Can you work these out from the model? Positions are in its coordinate system, mm. Face numbers are marked on the shaded views. A direction names the side the tool comes from. Give positions to 0.01 mm unless a question says otherwise; leave off trailing zeros. Loops run counter-clockwise (first coordinate to the right, second up) from the corner with the lowest first, then second, coordinate; pieces in that order, holes last. Notation, with made-up numbers: (37, 3.5) - (84, 3.5) arc R25 cw to (84, 27.5) - close; hole circle Ø2 at (77, 54). An arc over 180 degrees is marked (long way). Answer as a JSON object with one key per item and string values. Group by question number.
Item 1: Please list where these lines run through material, in increasing order: L1, parallel to Z at x = 0, y = 1; L2, parallel to X at y = -0.5, z = 1.
Item 2: Which directions (+Z, -Z, +X, -X, +Y, -Y) give clear straight access to the entire face, cutting with the end or side of a thin tool? Please do the marked faces 1 and 2.
Item 3: Suppose I cut it at C-C on y = 12. Write out the boundary of the cut face in (x, z), and give its area (3 significant figures).
Item 4: Will these pins go through, and if not, where does the flat tip stop? pin 1 (2 mm diameter, centred on y = 5, z = -2, fed in from -X); pin 2 (2 mm diameter, centred on y = 6, z = 1.5, fed in from +X); pin 3 (1 mm diameter, centred on x = 1.5, z = -2, fed in from -Y).
Item 5: Suppose I cut it at A-A on y = 7.75. Write out the boundary of the cut face in (x, z), and give its area (3 significant figures).
Item 6: Suppose I cut it at B-B on y = -6.75. Write out the boundary of the cut face in (x, z).
Item 7: Thinking about a two-plate mould opening in Z: for the marked faces 3, 4 and 5, which applies, pulls with the +Z half, pulls with the -Z half, needs draft (parallel to the pull), parting line crosses it, or undercut?
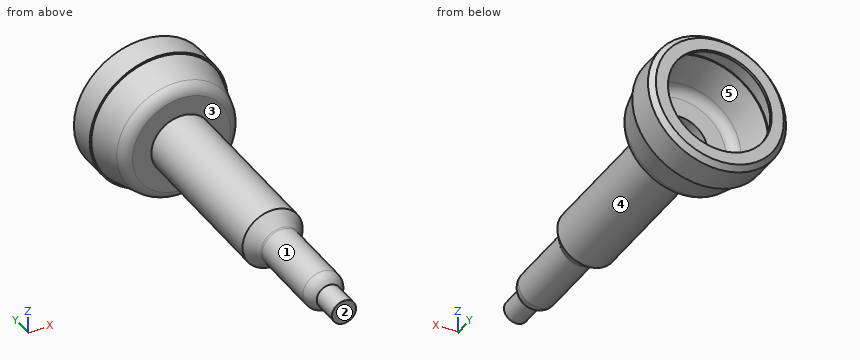
from build123d import *

# Parameters (mm, degrees)
BOSS_EXTRUDE1_DEPTH      = 7
BOSS_EXTRUDE1_DEPTH_BACK = 5
SKETCH2_R                = 1.4
SKETCH3_OUTSIDE_W        = 18.066
SKETCH3_OUTSIDE_H        = 18.066
SKETCH3_OUTSIDE_R        = 0.875
CUT_EXTRUDE1_DEPTH       = 2
FILLET1_R                = 1


with BuildPart() as part:
    # Sketch1 → Revolve2 (revolve)
    with BuildSketch(Plane.XY):
        with BuildLine():
            Line((-3.755778652, 14.546362803), (-4.55, 14.546362803))
            Line((-4.55, 14.546362803), (-4.8, 14.296362803))
            Line((-4.8, 14.296362803), (-4.8, 12.499997602))
            Line((-4.8, 12.499997602), (-4.726187471, 12.499997602))
            Line((-4.726187471, 12.499997602), (-4.085093395, 10.107402835))
            ThreePointArc((-4.085093395, 10.107402835), (-3.828996553, 9.665101687), (-3.348994918, 9.489561582))
            Line((-3.348994918, 9.489561582), (-2, 9.489561582))
            Line((-2, 9.489561582), (-2, -2.631922723))
            Line((-2, -2.631922723), (-1.256169591, -3.694222639))
            ThreePointArc((-1.256169591, -3.694222639), (-1.22925661, -3.748796766), (-1.22, -3.808937926))
            Line((-1.22, -3.808937926), (-1.22, -4.710135178))
            ThreePointArc((-1.22, -4.710135178), (-1.161421356, -4.851556534), (-1.02, -4.910135178))
            Line((-1.02, -4.910135178), (0, -4.910135178))
            Line((0, -4.910135178), (0, -5.090135178))
            Line((0, -5.090135178), (-1.2, -5.090135178))
            ThreePointArc((-1.2, -5.090135178), (-1.341421356, -5.031556534), (-1.4, -4.890135178))
            Line((-1.4, -4.890135178), (-1.4, -3.865691708))
            ThreePointArc((-1.4, -3.865691708), (-1.40925661, -3.805550548), (-1.436169591, -3.750976421))
            Line((-1.436169591, -3.750976421), (-2.18, -2.688676505))
            Line((-2.18, -2.688676505), (-2.18, 9.311323495))
            Line((-2.18, 9.311323495), (-3.548994918, 9.311323495))
            ThreePointArc((-3.548994918, 9.311323495), (-4.027869138, 9.577238986), (-4.280340775, 10.063335313))
            Line((-4.280340775, 10.063335313), (-4.879652854, 12.299997602))
            Line((-4.879652854, 12.299997602), (-5, 12.299997602))
            Line((-5, 12.299997602), (-5, 14.379205516))
            Line((-5, 14.379205516), (-4.632842712, 14.746362803))
            Line((-4.632842712, 14.746362803), (-3.755778652, 14.746362803))
            Line((-3.755778652, 14.746362803), (-3.755778652, 14.546362803))
        make_face()
    revolve(axis=Axis((0, 14.5, 0), (0, -1, 0)))

    # Sketch2 → Boss-Extrude1 (add, two sides: drawn at the far end of the back side and taken through both)
    with BuildSketch(Plane.XZ.offset(5.090135178).offset(-BOSS_EXTRUDE1_DEPTH_BACK)):
        with Locations(Location((0, 0, 0), (0, 0, 180))):
            Circle(SKETCH2_R)
    extrude(amount=BOSS_EXTRUDE1_DEPTH + BOSS_EXTRUDE1_DEPTH_BACK)

    # Sketch3 outside → Cut-Extrude1 (cut)
    with BuildSketch(Plane.XZ.offset(12.090135178)):
        Rectangle(SKETCH3_OUTSIDE_W, SKETCH3_OUTSIDE_H)
        Circle(SKETCH3_OUTSIDE_R, mode=Mode.SUBTRACT)
    extrude(amount=-CUT_EXTRUDE1_DEPTH, mode=Mode.SUBTRACT)

    # Fillet1
    # the kernel refuses this fillet: 1 mm, written as the material it takes off along each edge
    with BuildSketch(Plane(origin=(0, -10.090135178, 0), x_dir=(-1, 0, 0), z_dir=(0, 0, -1))) as fillet1_piece_1:
        with BuildLine():
            CenterArc((0.4, 0.879985795), FILLET1_R, 298.359350028, 61.640649972)
            Line((0.875, 0), (0.8845, -0.017599716))
            ThreePointArc((0.8845, -0.017599716), (1.1375, -0.02), (1.4, -0.02))
            Line((1.4, -0.02), (1.42, 0))
            Line((1.42, 0), (1.42, 0.879985795))
            Line((1.42, 0.879985795), (1.4, 0.879985795))
        make_face()
    revolve(axis=Axis((0, -10.090135178, 0), (0, 1, 0)), mode=Mode.SUBTRACT)


solid = part.part
Worked out:
{
 "1": {"L1": "z = -2.18 to -2, 2 to 2.18", "L2": "x = -1.94 to -1.73, -0.98 to 0.98, 1.73 to 1.94"},
 "2": {"face 1": "-Y", "face 2": "+Z, -Z, +X, -X, -Y"},
 "3": {"outline": "circle Ø9.6 at (0, 0); hole circle Ø9.18 at (0, 0)", "area": "6.11 mm2"},
 "4": {"pin 1": "stops at x = -1.94", "pin 2": "stops at x = 2.12", "pin 3": "stops at y = -2.95"},
 "5": {"outline": "circle Ø4.36 at (0, 0); hole circle Ø4 at (0, 0)", "area": "2.36 mm2"},
 "6": {"outline": "circle Ø2.8 at (0, 0)"},
 "7": {"face 3": "needs draft", "face 4": "parting line crosses it", "face 5": "undercut"}
}
